from build123d import *

# Parameters (mm, degrees)
SKETCH_1_W                = 60
SKETCH_1_H                = 60
EXTRUDE_1_DEPTH           = 6
HOLE_WIZARD_M3_1_D        = 2.5
HOLE_WIZARD_1_D           = 4
HOLE_WIZARD_1_CBORE_D     = 8
HOLE_WIZARD_1_CBORE_DEPTH = 4.8


with BuildPart() as part:
    # 草图1 → 凸台-拉伸1 (new body)
    with BuildSketch(Plane.XY):
        Rectangle(SKETCH_1_W, SKETCH_1_H)
    extrude(amount=EXTRUDE_1_DEPTH)

    # M3 螺纹孔1 (through all)
    with Locations(Plane(origin=(-25, 25, 6), x_dir=(1, 0, 0), z_dir=(0, 0, 1))):
        with Locations((0, 0), (50, 0), (50, -50), (0, -50)):
            Hole(HOLE_WIZARD_M3_1_D / 2)

    # 孔1 (through all)
    with Locations(Plane(origin=(-12.7, 12.7, 6), x_dir=(1, 0, 0), z_dir=(0, 0, 1))):
        with Locations((0, 0), (25.4, 0), (25.4, -25.4), (0, -25.4)):
            CounterBoreHole(HOLE_WIZARD_1_D / 2, HOLE_WIZARD_1_CBORE_D / 2, HOLE_WIZARD_1_CBORE_DEPTH)


solid = part.part
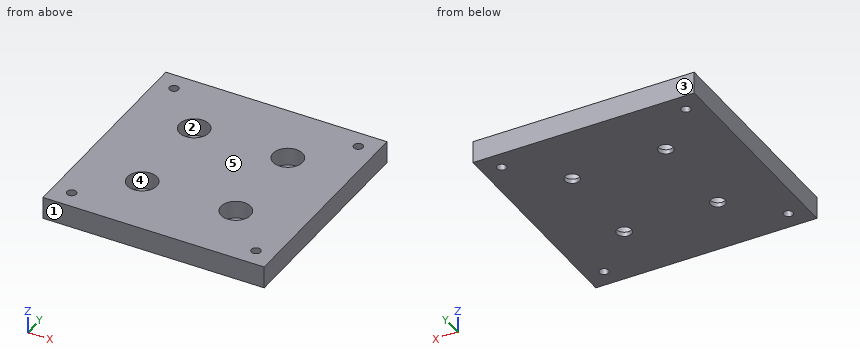
Source: CAD feature listing. Evaluate the final solid. Frame: model axes, mm. Face numbers are marked on the shaded views. A direction names the side the tool comes from. Coordinates: 2 decimals unless noted, no trailing zeros. Loops run counter-clockwise (first coordinate to the right, second up) from the corner with the lowest first, then second, coordinate; pieces in that order, holes last. Notation, with made-up numbers: M -15,23 L 37,23 A31 cw 37,57 Z; hole C -13.5,68.5 d10. An arc over 180 degrees is marked long. Answer in a Markdown table with one row per item.
Q1. Draft query along Y for the marked faces 1, 2 and 3. Return one class per face: pulls with the +Y half, pulls with the -Y half, needs draft (parallel to the pull), parting line crosses it, or undercut.
Answers below:
| item | result |
|---|---|
| face 1 | pulls with the -Y half |
| face 2 | undercut |
| face 3 | pulls with the +Y half |
Q2. Section D-D on x = -25. Return the cut outline in (y, z), plus the area to 3 significant figures.
Answers below:
| item | result |
|---|---|
| outline | M -30,0 L -26.25,0 L -26.25,6 L -30,6 Z; M -23.75,0 L 23.75,0 L 23.75,6 L -23.75,6 Z; M 26.25,0 L 30,0 L 30,6 L 26.25,6 Z |
| area | 330 mm^2 |
Q3. Ray query, probe 1 along Y at (x, z) = (-12.7, 0.4); probe 2 along Y at (x, z) = (-25, 2.6); probe 3 along X at (y, z) = (-10, 2.35). Return the intervals inside material, ascending. Write a range as from..to.
Answers below:
| item | result |
|---|---|
| probe 1 | y = -30..-14.7, -10.7..10.7, 14.7..30 |
| probe 2 | y = -30..-26.25, -23.75..23.75, 26.25..30 |
| probe 3 | x = -30..-15.65, -9.75..9.75, 15.65..30 |
Q4. First-contact query: pin 1 (6.5 mm diameter, centred on x = 12.7, y = -12.7, fed in from -Z); pin 2 (2.5 mm diameter, centred on x = 11, y = 14, fed in from +Z). Flat tips, straight axial feed; report the tip coordinate or a pass-through.
Answers below:
| item | result |
|---|---|
| pin 1 | stops at z = 0 |
| pin 2 | stops at z = 1.2 |
Q5. Set-up query: the marked faces 4 and 5. Return all of +Z, -Z, +X, -X, +Y, -Y with unobstructed straight access to the full face (end or side cutting, diameter ignored); none if empty.
Answers below:
| item | result |
|---|---|
| face 4 | +Z |
| face 5 | +Z, +X, -X, +Y, -Y |
Q6. Section A-A on x = 12.7. Return the cut outline in (y, z).
Answers below:
| item | result |
|---|---|
| outline | M -30,0 L -14.7,0 L -14.7,1.2 L -16.7,1.2 L -16.7,6 L -30,6 Z; M -10.7,0 L 10.7,0 L 10.7,1.2 L 8.7,1.2 L 8.7,6 L -8.7,6 L -8.7,1.2 L -10.7,1.2 Z; M 14.7,0 L 30,0 L 30,6 L 16.7,6 L 16.7,1.2 L 14.7,1.2 Z |
Q7. Section C-C on z = 2.25. State how many separate pieces and enclosed holes the cut face has, plus the area to 3 significant figures.
Answers below:
| item | result |
|---|---|
| separate pieces | 1 |
| enclosed holes | 8 |
| area | 3,380 mm^2 |
